Check sheet for the modelled part. Datum: model origin and axes. Units: mm. A direction names the side the tool comes from. Coordinates: 2 decimals unless noted, no trailing zeros. Order: outer loops, then holes, each group sorted by start corner. A loop starts at its lowest first (then second) coordinate and runs counter-clockwise, first axis right, second up.
from build123d import *

# Parameters (mm, degrees)
SKETCH1_W           = 14
SKETCH1_H           = 2
BOSS_EXTRUDE1_DEPTH = 3
CHAMFER1_SIZE       = 0.5
SKETCH2_W           = 2
SKETCH2_H           = 1
BOSS_EXTRUDE2_DEPTH = 2
SKETCH3_R           = 0.5
CUT_EXTRUDE1_DEPTH  = 2


with BuildPart() as part:
    # Sketch1 → Boss-Extrude1 (new body)
    with BuildSketch(Plane(origin=(0, 0, 0), x_dir=(1, 0, 0), z_dir=(0, 1, 0))):
        Rectangle(SKETCH1_W, SKETCH1_H)
    extrude(amount=BOSS_EXTRUDE1_DEPTH)

    # Chamfer1
    chamfer1_edges = [part.edges().sort_by_distance(p)[0] for p in [
        (0, 0, -1),
        (7, 1.5, -1),
        (0, 3, -1),
    ]]
    chamfer(chamfer1_edges, length=CHAMFER1_SIZE)

    # Sketch2 → Boss-Extrude2 (add)
    with BuildSketch(Plane.ZY.offset(7)):
        with Locations((0, 1.5)):
            Rectangle(SKETCH2_W, SKETCH2_H)
    extrude(amount=BOSS_EXTRUDE2_DEPTH)

    # Sketch3 → Cut-Extrude1 (cut)
    with BuildSketch(Plane(origin=(0, 2, 0), x_dir=(1, 0, 0), z_dir=(0, 1, 0))):
        with Locations(Location((-8, 0, 0), (0, 0, 270))):
            Circle(SKETCH3_R)
        with BuildLine():
            ThreePointArc((-9, 0), (-8.707106781, 0.707106781), (-8, 1))
            Line((-8, 1), (-9, 1))
            Line((-9, 1), (-9, 0))
        make_face()
        with BuildLine():
            Line((-9, -1), (-8, -1))
            ThreePointArc((-8, -1), (-8.707106781, -0.707106781), (-9, 0))
            Line((-9, 0), (-9, -1))
        make_face()
    extrude(amount=-CUT_EXTRUDE1_DEPTH, mode=Mode.SUBTRACT)


with BuildPart() as body_2:
    # Mirror1: mirrored copy
    add(part.part.mirror(Plane(origin=(-7, 3, -1), x_dir=(1, 0, 0), z_dir=(0, 0, 1))))


solid = body_2.part
(1) Cross-section at A-A (z = -1.85). Enter the section's corners in (x, y), and give its area (3 significant figures).
Filled in:
outline: (-8.99, 1) - (-8.48, 1) - (-8.48, 2) - (-8.99, 2) - close; (-7.52, 1) - (-7, 1) - (-7, 0) - (7, 0) - (7, 3) - (-7, 3) - (-7, 2) - (-7.52, 2) - close
area: 43.0 mm2
(2) Go/stop test with flat-tipped pins: P1, Ø0.6, axis at x = -7.5, z = -2.5, coming from the -Y side; P2, Ø0.5, axis at y = 0.5, z = -2, coming from the -X side; P3, Ø0.6, axis at x = -8.5, z = -1.5, coming from the +Y side. Record where each tip stops, or that it passes through.
Filled in:
P1: stops at y = 1
P2: stops at x = -7
P3: stops at y = 2
(3) Thickness scan on probe 1 along X at (y, z) = (1.65, -2); probe 2 along X at (y, z) = (2.8, -2); probe 3 along Y at (x, z) = (-7.25, -1.6). Record the ranges inside material, lowest first.
Filled in:
probe 1: x = -9 to -8.5, -7.5 to 7
probe 2: x = -7 to 7
probe 3: y = 1 to 2
(4) Cross-section at C-C (y = 2.3). Enter the section's corners in (x, z).
Filled in:
outline: (-7, -3) - (7, -3) - (7, -1.5) - (6.5, -1) - (-7, -1) - close
(5) Release check for a two-part mould opening along X. For faces 1 (the flat face through (-7.5, 1, -1.5)), 2 (the cylindrical face through (-8.488, 1.507, -1.892)), 3 (the flat face through (7, 1, -2)), 4 (the flat face through (-7, 2.5, -2)) record: +X half, -X half, draft (parallel to the pull), parting line (faces both ways), or undercut.
Filled in:
face 1: draft
face 2: undercut
face 3: +X half
face 4: -X half
(6) Tool access check on faces 5 (the flat face through (-7.5, 2, -1.5)), 6 (the flat face through (-7, 0.5, -2)), 7 (the flat face through (-1, 1, -3)). Record the directions out of +Z, -Z, +X, -X, +Y, -Y that give a thin tool (end or side, any length) a straight path to the whole face; none if there is none.
Filled in:
face 5: +Z, -Z, -X, +Y
face 6: +Z, -Z, -X, -Y
face 7: -Z, +X, -X, +Y, -Y
(7) Cross-section at B-B (x = 3). Enter the section's corners in (y, z).
Filled in:
outline: (0, -3) - (3, -3) - (3, -1.5) - (2.5, -1) - (0.5, -1) - (0, -1.5) - close
(8) Cross-section at D-D (z = -2.75). Enter the section's corners in (x, y).
Filled in:
outline: (-8.66, 1) - (-7, 1) - (-7, 0) - (7, 0) - (7, 3) - (-7, 3) - (-7, 2) - (-8.66, 2) - close
